```python
from build123d import *

# Parameters (mm, degrees)
BOSS_EXTRUDE1_DEPTH      = 80
BOSS_EXTRUDE2_DEPTH      = 80
BOSS_EXTRUDE3_DEPTH      = 2.5
BOSS_EXTRUDE6_START      = -2.5
BOSS_EXTRUDE6_DEPTH      = 2.5
BOSS_EXTRUDE7_REACH      = 202.922
BOSS_EXTRUDE7_END_RADIUS = 60
BOSS_EXTRUDE7_START      = 75
SKETCH10_W               = 80
SKETCH10_H               = 4.1
SKETCH11_R               = 2.05
CUT_EXTRUDE3_DEPTH       = 4.1
BOSS_EXTRUDE5_REACH      = 205.768
BOSS_EXTRUDE5_START      = -75
SKETCH7_W                = 80
SKETCH7_H                = 4.1
SKETCH8_R                = 2.05
CUT_EXTRUDE2_DEPTH       = 12.5


with BuildPart() as part:
    # Sketch1 → Boss-Extrude1 (new body)
    with BuildSketch(Plane.XY):
        with BuildLine():
            Line((29.047375097, 15), (70, 15))
            Line((70, 15), (70, 0))
            Line((70, 0), (-70, 0))
            Line((-70, 0), (-70, 15))
            Line((-70, 15), (-29.047375097, 15))
            ThreePointArc((-29.047375097, 15), (0, 7.5), (29.047375097, 15))
        make_face()
    extrude(amount=BOSS_EXTRUDE1_DEPTH)

    # Sketch2 → Boss-Extrude2 (add)
    with BuildSketch(Plane(origin=(0, 0, 0), x_dir=(-1, 0, 0), z_dir=(0, 0, -1))):
        with BuildLine():
            Line((-60, 67.5), (-57.5, 67.5))
            ThreePointArc((-57.5, 67.5), (0, 10), (57.5, 67.5))
            Line((57.5, 67.5), (60, 67.5))
            ThreePointArc((60, 67.5), (0, 7.5), (-60, 67.5))
        make_face()
    extrude(amount=-BOSS_EXTRUDE2_DEPTH)

    # Sketch3 → Boss-Extrude3 (add)
    with BuildSketch(Plane(origin=(0, 0, 0), x_dir=(-1, 0, 0), z_dir=(0, 0, -1))):
        with BuildLine():
            Line((-57.5, 67.5), (-48.75, 67.5))
            ThreePointArc((-48.75, 67.5), (0, 18.75), (48.75, 67.5))
            Line((48.75, 67.5), (57.5, 67.5))
            ThreePointArc((57.5, 67.5), (0, 10), (-57.5, 67.5))
        make_face()
    extrude(amount=-BOSS_EXTRUDE3_DEPTH)

    # Sketch9 → Boss-Extrude6 (add)
    with BuildSketch(Plane.XY.offset(80).offset(BOSS_EXTRUDE6_START)):
        with BuildLine():
            Line((-57.5, 67.5), (-15, 67.5))
            ThreePointArc((-15, 67.5), (0, 52.5), (15, 67.5))
            Line((15, 67.5), (57.5, 67.5))
            ThreePointArc((57.5, 67.5), (0, 10), (-57.5, 67.5))
        make_face()
    extrude(amount=BOSS_EXTRUDE6_DEPTH)

    # Boss-Extrude7: up to this cylinder (the profile starts outside it)
    boss_extrude7_end = Plane(origin=(0, 67.5, 40), z_dir=(0, 0, -1)) * Cylinder(BOSS_EXTRUDE7_END_RADIUS, 526.844, mode=Mode.PRIVATE)
    # Sketch10 → Boss-Extrude7 (add, up to the surface)
    with BuildSketch(Plane(origin=(0, 0, 0), x_dir=(0, 0, -1), z_dir=(1, 0, 0)).offset(BOSS_EXTRUDE7_START), mode=Mode.PRIVATE) as boss_extrude7_sk1:
        with Locations((-40, 65.45)):
            Rectangle(SKETCH10_W, SKETCH10_H)
    boss_extrude7_tool1 = extrude(boss_extrude7_sk1.sketch, amount=-BOSS_EXTRUDE7_REACH, mode=Mode.PRIVATE) - boss_extrude7_end
    boss_extrude7 = boss_extrude7_tool1.solids().sort_by_distance((75, 65.45, 40))[0]
    add(boss_extrude7)

    # Sketch11 → Cut-Extrude3 (cut)
    with BuildSketch(Plane(origin=(0, 67.5, 0), x_dir=(1, 0, 0), z_dir=(0, 1, 0))):
        with Locations(Location((67.5, -70, 0), (0, 0, 270))):
            Circle(SKETCH11_R)
        with Locations(Location((67.5, -50, 0), (0, 0, 270))):
            Circle(SKETCH11_R)
        with Locations(Location((67.5, -30, 0), (0, 0, 270))):
            Circle(SKETCH11_R)
        with Locations(Location((67.5, -10, 0), (0, 0, 270))):
            Circle(SKETCH11_R)
    cut_extrude3 = extrude(amount=-CUT_EXTRUDE3_DEPTH, mode=Mode.SUBTRACT)

    # Mirror3: Boss-Extrude7, Cut-Extrude3 across plane
    add(boss_extrude7.mirror(Plane(origin=(0, 0, 0), x_dir=(0, 0, 1), z_dir=(1, 0, 0))))
    add(cut_extrude3.mirror(Plane(origin=(0, 0, 0), x_dir=(0, 0, 1), z_dir=(1, 0, 0))), mode=Mode.SUBTRACT)

    # Sketch7 → Boss-Extrude5 (add, up to next)
    with BuildSketch(Plane(origin=(0, 0, 0), x_dir=(0, 0, -1), z_dir=(1, 0, 0)).offset(BOSS_EXTRUDE5_START), mode=Mode.PRIVATE) as boss_extrude5_sk1:
        with Locations((-40, 65.45)):
            Rectangle(SKETCH7_W, SKETCH7_H)
    boss_extrude5_tool1 = extrude(boss_extrude5_sk1.sketch, amount=BOSS_EXTRUDE5_REACH, mode=Mode.PRIVATE) - part.part
    add(boss_extrude5_tool1.solids().sort_by_distance((-75, 65.45, 40))[0])

    # Sketch8 → Cut-Extrude2 (cut)
    with BuildSketch(Plane(origin=(0, 67.5, 0), x_dir=(1, 0, 0), z_dir=(0, 1, 0))):
        with Locations(Location((-67.5, -10, 0), (0, 0, 270))):
            Circle(SKETCH8_R)
        with Locations(Location((-67.5, -30, 0), (0, 0, 270))):
            Circle(SKETCH8_R)
        with Locations(Location((-67.5, -50, 0), (0, 0, 270))):
            Circle(SKETCH8_R)
        with Locations(Location((-67.5, -70, 0), (0, 0, 270))):
            Circle(SKETCH8_R)
    cut_extrude2 = extrude(amount=-CUT_EXTRUDE2_DEPTH, mode=Mode.SUBTRACT)

    # Mirror2: Cut-Extrude2 across plane
    add(cut_extrude2.mirror(Plane(origin=(0, 0, 0), x_dir=(0, 0, 1), z_dir=(1, 0, 0))), mode=Mode.SUBTRACT)


solid = part.part
```
CAD build for the part. Positions are in the model's coordinates, mm. A direction names the side the tool comes from. Coordinates: 2 decimals unless noted, no trailing zeros. Loops run counter-clockwise (first coordinate to the right, second up) from the corner with the lowest first, then second, coordinate; pieces in that order, holes last. Notation, with made-up numbers: (11, 78.5) - (68, 78.5) arc R22 ccw to (68, 107.5) - close; hole circle Ø5 at (59, 6.25). An arc over 180 degrees is marked (long way). Return JSON: item names as keys, results as strings.
1. 3-axis set-ups, long thin cutter, end or side, ignore diameter. For faces 4 (the flat face through (49, 15, 39)), 5 (the cylindrical face through (68.9, 65.5, 48.5)), 6 (the flat face through (-70, 7, 39)): which of +Z, -Z, +X, -X, +Y, -Y reach the whole face in a straight line?
Result:
{"face 4": "+Z, -Z, +X", "face 5": "+Y", "face 6": "+Z, -Z, -X, -Y"}
2. Drop flat-ended pins along their axis: pin 1 (8 mm diameter, centred on y = 16, z = 50, fed in from +X); pin 2 (12 mm diameter, centred on x = 38.5, z = 39.5, fed in from +Y); pin 3 (2 mm diameter, centred on x = 0, y = 31, fed in from -Z). Give the stop position or say it passes through.
Result:
{"pin 1": "stops at x = 70", "pin 2": "stops at y = 31.09", "pin 3": "stops at z = 77.5"}
3. Band-saw the part on B-B (x = -67.5). Give the cut face in (y, z).
Result:
{"outline": "(0, 0) - (15, 0) - (15, 80) - (0, 80) - close; (63.4, 0) - (67.5, 0) - (67.5, 7.95) - (63.4, 7.95) - close; (63.4, 12.05) - (67.5, 12.05) - (67.5, 27.95) - (63.4, 27.95) - close; (63.4, 32.05) - (67.5, 32.05) - (67.5, 47.95) - (63.4, 47.95) - close; (63.4, 52.05) - (67.5, 52.05) - (67.5, 67.95) - (63.4, 67.95) - close; (63.4, 72.05) - (67.5, 72.05) - (67.5, 80) - (63.4, 80) - close"}
4. Probe L1, parallel to X at y = 65.95, z = 10; L2, parallel to X at y = 64, z = 10; L3, parallel to Z at x = 16.5, y = 18. List the from-to ranges inside material, lowest first. Write a range as from..to.
Result:
{"L1": "x = -75..-69.55, -65.45..-57.48, 57.48..65.45, 69.55..75", "L2": "x = -75..-69.55, -65.45..-57.39, 57.39..65.45, 69.55..75", "L3": "z = 0..2.5, 77.5..80"}
5. Mould opens along X. For faces 1 (the flat face through (70, 8, 39)), 2 (the flat face through (-68, 63.4, 41)), 3 (the cylindrical face through (1.264, 10.014, 39.475)) say: released by +X, released by -X, zero draft, split by the parting line, or undercut.
Result:
{"face 1": "released by +X", "face 2": "zero draft", "face 3": "undercut"}
6. Band-saw the part on C-C (x = -40). Give the cut face in (y, z).
Result:
{"outline": "(0, 0) - (15, 0) - (15, 80) - (0, 80) - close; (22.78, 0) - (39.63, 0) - (39.63, 2.5) - (26.19, 2.5) - (26.19, 77.5) - (67.5, 77.5) - (67.5, 80) - (22.78, 80) - close"}
7. Band-saw the part on A-A (z = 30). Give the cut face in (x, y), and give its area (3 significant figures).
Result:
{"outline": "(-75, 63.4) - (-69.55, 63.4) - (-69.55, 67.5) - (-75, 67.5) - close; (-70, 0) - (70, 0) - (70, 15) - (29.05, 15) arc R60 ccw to (59.86, 63.4) - (65.45, 63.4) - (65.45, 67.5) - (57.5, 67.5) arc R57.5 cw to (-57.5, 67.5) - (-65.45, 67.5) - (-65.45, 63.4) - (-59.86, 63.4) arc R60 ccw to (-29.05, 15) - (-70, 15) - close; (69.55, 63.4) - (75, 63.4) - (75, 67.5) - (69.55, 67.5) - close", "area": "2,360 mm2"}
8. Band-saw the part on D-D (y = 33). Give the cut face in (x, z), and give its area (3 significant figures).
Result:
{"outline": "(-49.09, 0) - (-34.44, 0) - (-34.44, 2.5) - (-46, 2.5) - (-46, 77.5) - (46, 77.5) - (46, 2.5) - (34.44, 2.5) - (34.44, 0) - (49.09, 0) - (49.09, 80) - (-49.09, 80) - close", "area": "782 mm2"}
